```python
from build123d import *

# Parameters (mm, degrees)
SZKIC1_R                    = 4.635188213
SZKIC1_R_2                  = 3.000000079
SZKIC1_R_3                  = 5.522620658
DODANIE_WYCI_GNI_CIE1_DEPTH = 5
SZKIC2_W                    = 1.618528634
SZKIC2_H                    = 7.505645785
SZKIC2_W_2                  = 0.651830256
SZKIC2_H_2                  = 5.051684483
WYTNIJ_WYCI_GNI_CIE3_DEPTH  = 6


with BuildPart() as part:
    # Szkic1 → Dodanie-wyciągnięcie1 (new body)
    with BuildSketch(Plane.XY):
        with BuildLine():
            ThreePointArc((182.852037835, 2.527386464), (184.886505162, 4.714718212), (187.7624, 5.522620658))
            ThreePointArc((187.7624, 5.522620658), (93.841201508, 13.541760303), (0, 4.635188213))
            ThreePointArc((0, 4.635188213), (2.197225531, 4.081319607), (3.869348656, 2.552079691))
            ThreePointArc((3.869348656, 2.552079691), (4.951964009, 2.784051377), (6.035181021, 3.013197121))
            ThreePointArc((6.035181021, 3.013197121), (93.702955413, 12.084887853), (181.353491517, 2.8481265))
            ThreePointArc((181.353491517, 2.8481265), (182.102909488, 2.688433069), (182.852037835, 2.527386464))
        make_face()
        with BuildLine():
            ThreePointArc((0, -4.635188213), (93.841201508, -13.541760303), (187.7624, -5.522620658))
            ThreePointArc((187.7624, -5.522620658), (184.886505162, -4.714718212), (182.852037835, -2.527386464))
            ThreePointArc((182.852037835, -2.527386464), (182.102909488, -2.688433069), (181.353491517, -2.8481265))
            ThreePointArc((181.353491517, -2.8481265), (93.702955413, -12.084887853), (6.035181021, -3.013197121))
            ThreePointArc((6.035181021, -3.013197121), (4.951964009, -2.784051377), (3.869348656, -2.552079691))
            ThreePointArc((3.869348656, -2.552079691), (2.197225531, -4.081319607), (0, -4.635188213))
        make_face()
        Circle(SZKIC1_R)
        Circle(SZKIC1_R_2, mode=Mode.SUBTRACT)
        with BuildLine():
            ThreePointArc((4.561393731, -0.823806409), (4.303032237, -1.723044787), (3.869348656, -2.552079691))
            ThreePointArc((3.869348656, -2.552079691), (4.951964009, -2.784051377), (6.035181021, -3.013197121))
            ThreePointArc((6.035181021, -3.013197121), (4.853956333, -2.21760299), (4.561393731, -0.823806409))
        make_face()
        with BuildLine():
            ThreePointArc((6.035181021, 3.013197121), (4.951964009, 2.784051377), (3.869348656, 2.552079691))
            ThreePointArc((3.869348656, 2.552079691), (4.303032237, 1.723044787), (4.561393731, 0.823806409))
            ThreePointArc((4.561393731, 0.823806409), (4.853956333, 2.21760299), (6.035181021, 3.013197121))
        make_face()
        with BuildLine():
            ThreePointArc((181.353491517, -2.8481265), (182.102909488, -2.688433069), (182.852037835, -2.527386464))
            ThreePointArc((182.852037835, -2.527386464), (182.576004096, -1.897534311), (182.380388165, -1.238259886))
            ThreePointArc((182.380388165, -1.238259886), (182.204390831, -2.258445368), (181.353491517, -2.8481265))
        make_face()
        with Locations((187.7624, 0)):
            Circle(SZKIC1_R_3)
        with Locations((187.7624, 0)):
            Circle(SZKIC1_R_2, mode=Mode.SUBTRACT)
        with BuildLine():
            ThreePointArc((182.380388165, 1.238259886), (182.576004096, 1.897534311), (182.852037835, 2.527386464))
            ThreePointArc((182.852037835, 2.527386464), (182.102909488, 2.688433069), (181.353491517, 2.8481265))
            ThreePointArc((181.353491517, 2.8481265), (182.204390831, 2.258445368), (182.380388165, 1.238259886))
        make_face()
    extrude(amount=DODANIE_WYCI_GNI_CIE1_DEPTH)

    # Szkic2 → Wytnij-wyciągnięcie3 (cut, through all)
    with BuildSketch(Plane.XY):
        with Locations((193.638606269, 0.381285041)):
            Rectangle(SZKIC2_W, SZKIC2_H)
        with Locations((-4.682734605, -0.038745932)):
            Rectangle(SZKIC2_W_2, SZKIC2_H_2)
    extrude(amount=WYTNIJ_WYCI_GNI_CIE3_DEPTH, mode=Mode.SUBTRACT)


solid = part.part
```
CAD build for the part. Positions are in the model's coordinates, mm. A direction names the side the tool comes from. Round coordinates to 2 decimals unless told otherwise and drop trailing zeros. Write each loop counter-clockwise with the first axis right and the second up, starting at its lowest first coordinate (ties: lowest second). Pieces come first, ordered by that corner, then holes. Notation, with made-up numbers: (-31.75, 75) -> (-2.75, 75) arc R27 cw to (-2.75, 97) -> close; hole circle Ø2 at (9.25, 0). An arc over 180 degrees is marked (long way). Answer in a Markdown table with one row per item. Add a question column.
Item 1: Saw through at A-A, the plane z = 2.05. Write the cut outline in (x, y).
Item 2: Saw through at C-C, the plane x = 79. Write the cut outline in (y, z), then the cut area to 3 significant figures.
Item 3: Mould opens along Y. For faces 1 (the face through (190.83, 4.59, 2.46)), 2 (the face through (101, 13, 5)), 3 (the face through (92.467, 12.084, 2.465)), 4 (the face through (190.76, -4.64, 2.46)) say: pulls with the +Y half, pulls with the -Y half, needs draft (parallel to the pull), parting line crosses it, or undercut.
Item 4: Drill centre lines: line 1 (X direction, y = 0.75, z = 0.35); line 2 (Y direction, x = 155.5, z = 0.2); line 3 (Y direction, x = 52, z = 1.15). Where is each one in solid material? Low to high. Write a range as from..to.
Item 5: Which spindle directions (+Z, -Z, +X, -X, +Y, -Y) get a long thin tool onto all of the face, cutting with end or side? Do faces 5 (the face through (94.94, -12.08, 2.46)), 6 (the face through (101, 13, 0)). Say none if no direction does.
Item 6: Drop flat-ended pins along their axis: pin 1 Ø1 at (x, z) = (128, 2) entering from +Y; pin 2 Ø5 at (x, y) = (0, 0) entering from +Z; pin 3 Ø3 at (x, z) = (156.5, 4) entering from +Y. Give the stop position or say it passes through.
Findings below:
| question | item | result |
|---|---|---|
| 1 | outline | (-4.36, -1.58) arc R4.64 ccw to (0, -4.64) arc R524.96 ccw to (187.76, -5.52) arc R5.52 ccw to (192.83, -2.2) -> (192.83, 2.2) arc R5.52 ccw to (187.76, 5.52) arc R524.96 ccw to (0, 4.64) arc R4.64 ccw to (-4.36, 1.58) -> close; hole circle Ø6 at (0, 0); hole (4.56, -0.82) arc R1.89 ccw to (6.04, -3.01) arc R424.28 ccw to (181.35, -2.85) arc R1.34 ccw to (182.38, -1.24) arc R5.52 cw to (182.38, 1.24) arc R1.34 ccw to (181.35, 2.85) arc R424.28 ccw to (6.04, 3.01) arc R1.89 ccw to (4.56, 0.82) arc R4.64 cw to start; hole circle Ø6 at (187.76, 0) |
| 2 | outline | (-13.26, 0) -> (-11.84, 0) -> (-11.84, 5) -> (-13.26, 5) -> close; (11.84, 0) -> (13.26, 0) -> (13.26, 5) -> (11.84, 5) -> close |
| 2 | area | 14.2 mm^2 |
| 3 | face 1 | pulls with the +Y half |
| 3 | face 2 | needs draft |
| 3 | face 3 | undercut |
| 3 | face 4 | pulls with the -Y half |
| 4 | line 1 | x = -4.36..-2.9, 2.9..4.57, 182.29..184.86, 190.67..192.83 |
| 4 | line 2 | y = -10.2..-7.5, 7.5..10.2 |
| 4 | line 3 | y = -11.67..-10.07, 10.07..11.67 |
| 5 | face 5 | +Z, -Z |
| 5 | face 6 | -Z, +X, -X, +Y, -Y |
| 6 | pin 1 | stops at y = 12.62 |
| 6 | pin 2 | passes through |
| 6 | pin 3 | stops at y = 10.26 |
